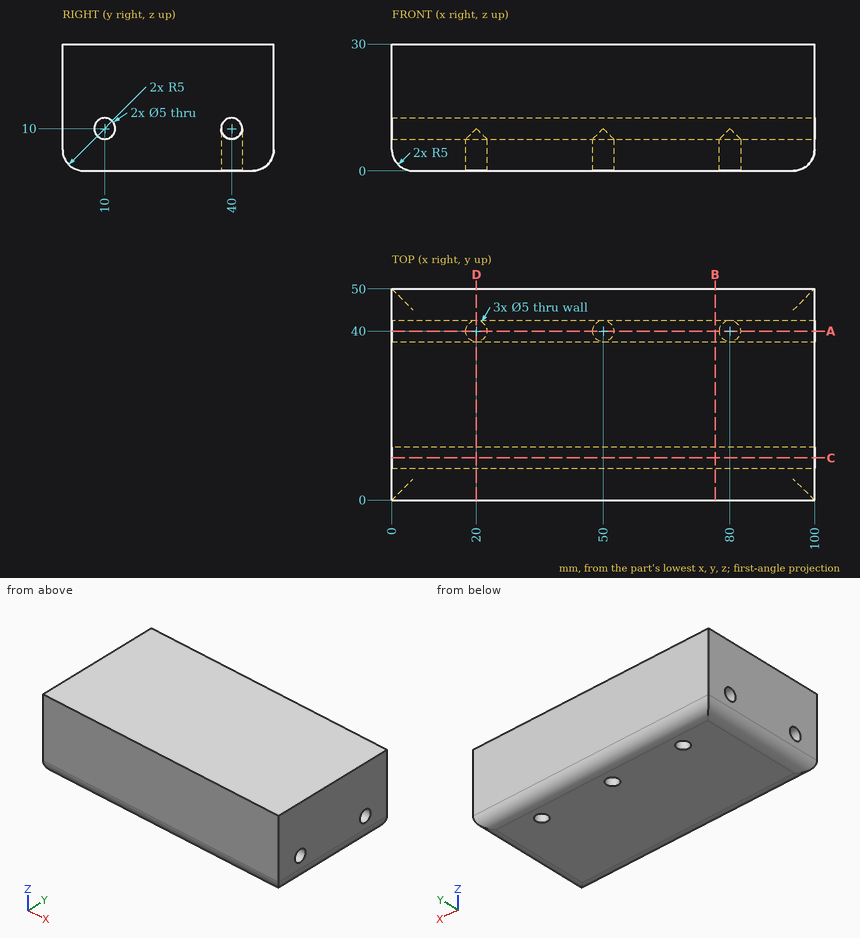
The drawing under review shows one solid part. Ordinate dimensions are in mm from its lowest x, y, z. Round coordinates to 2 decimals unless told otherwise and drop trailing zeros. Write each loop counter-clockwise with the first axis right and the second up, starting at its lowest first coordinate (ties: lowest second). Pieces come first, ordered by that corner, then holes. Notation, with made-up numbers: M 34,81.5 L 43,81.5 A22 ccw 43,103.5 Z; hole C 63.5,82 d4. An arc over 180 degrees is marked long. One line per item, written item: value. Start each with the question number.
(1) Wall thickness on line 1 (Z direction, x = 71, y = 40); line 2 (Y direction, x = 50, z = 5); line 3 (Y direction, x = 80, z = 4.25): over which ranges is each line inside the solid? List them lowest first.
(2) We need section D-D (x = 20). Give the boundary of the cut face in (y, z).
(3) We need section C-C (y = 10). Give the boundary of the cut face in (x, z).
(4) We need section B-B (x = 76.5). Give the boundary of the cut face in (y, z), and give its area (3 significant figures).
(5) We need section A-A (y = 40). Give the boundary of the cut face in (x, z).
Result:
1. line 1: 0 to 7.5, 12.5 to 30
1. line 2: 0 to 37.5, 42.5 to 50
1. line 3: 0.06 to 37.5, 42.5 to 49.94
2. outline: M 0,5 A5 ccw 5,0 L 37.5,0 L 37.5,10 A2.5 cw 42.5,10 L 42.5,0 L 45,0 A5 ccw 50,5 L 50,30 L 0,30 Z; hole C 10,10 d5
3. outline: M 0,5 A5 ccw 5,0 L 95,0 A5 ccw 100,5 L 100,7.5 L 0,7.5 Z; M 0,12.5 L 100,12.5 L 100,30 L 0,30 Z
4. outline: M 0,5 A5 ccw 5,0 L 45,0 A5 ccw 50,5 L 50,30 L 0,30 Z; hole C 10,10 d5; hole C 40,10 d5
4. area: 1,450 mm²
5. outline: M 0,5 A5 ccw 5,0 L 17.5,0 L 17.5,7.5 L 0,7.5 Z; M 0,12.5 L 100,12.5 L 100,30 L 0,30 Z; M 22.5,0 L 47.5,0 L 47.5,7.5 L 22.5,7.5 Z; M 52.5,0 L 77.5,0 L 77.5,7.5 L 52.5,7.5 Z; M 82.5,0 L 95,0 A5 ccw 100,5 L 100,7.5 L 82.5,7.5 Z
